Source: CAD feature listing. Evaluate the final solid. Frame: model axes, mm. Face numbers are marked on the shaded views. A direction names the side the tool comes from. Coordinates: 2 decimals unless noted, no trailing zeros. Loops run counter-clockwise (first coordinate to the right, second up) from the corner with the lowest first, then second, coordinate; pieces in that order, holes last. Notation, with made-up numbers: M 84.5,64 L 91.5,64 A22 ccw 91.5,75 Z; hole C -31,53.25 d6. An arc over 180 degrees is marked long. One line per question, with ' | ' between items. Start each with the question number.
1. Section query B-B, the plane x = 17.5. Output: boundary loops of the cut face in (y, z), and give its area (3 significant figures).
2. Section query A-A, the plane z = 3.5. Output: boundary loops of the cut face in (x, y), and give its area (3 significant figures).
3. Section query C-C, the plane y = 9.5. State how many separate pieces and enclosed holes the cut face has, and give its area (3 significant figures).
4. Ray query, probe 1 along Z at (x, y) = (17.5, 5.75); probe 2 along Z at (x, y) = (17.5, 2.1); probe 3 along X at (y, z) = (8, 3). Return the intervals inside material, ascending.
5. Mould query, pull axis X, two halves, no side actions, for the marked faces 1, 2, 3 and 4. Classes: pulls with the +X half, pulls with the -X half, needs draft (parallel to the pull), parting line crosses it, or undercut.
6. Access query for the marked faces 5 and 6. Directions: +Z, -Z, +X, -X, +Y, -Y. A direction counts if a zero-diameter tool reaches every point of the face in a straight line with its end or side. Return the directions, or none.
7. Section query D-D, the plane z = 22.5. Output: boundary loops of the cut face in (x, y).
8. Pin query (flat end, axial travel): P1, Ø12, axis at y = 15, z = 16.5, coming from the +X side; P2, Ø1.8, axis at x = 19, y = 8.5, coming from the +Z side; P3, Ø6, axis at x = 18, z = 9.5, coming from the +Y side. Return the tip coordinate at first contact, or that it passes through.
```python
from build123d import *

# Parameters (mm, degrees)
F0_W      = 20
F0_H      = 20
F0_R      = 2.75
F1_DEPTH  = 4
F2_W      = 20
F2_H      = 26
F3_DEPTH  = 3
F5_W      = 5
F5_H      = 9
F6_DEPTH  = 3
F4_R      = 1.4
F7_DEPTH  = 10
F9_DEPTH  = 3
F10_SIZE2 = 1.49999
F10_SIZE  = 2.99999


# Not quite as in the source:
# - a fillet or chamfer is up to 0.001 mm smaller than in the source, because OpenCascade refuses the exact size


with BuildPart() as f1:
    # F0 (on Top) → F1 (new body)
    with BuildSketch(Plane.XY):
        with Locations((10, 10)):
            Rectangle(F0_W, F0_H)
        with Locations((10, 10)):
            Circle(F0_R, mode=Mode.SUBTRACT)
    extrude(amount=F1_DEPTH)

    # F2 (on face) → F3 (join)
    with BuildSketch(Plane.XZ):
        with Locations((10, 13)):
            Rectangle(F2_W, F2_H)
    extrude(amount=-F3_DEPTH)

    # F5 (on face) → F6 (join)
    with BuildSketch(Plane.XY.offset(4)):
        with Locations((17.5, 7.5)):
            Rectangle(F5_W, F5_H)
    extrude(amount=F6_DEPTH)

    # F4 (on face) → F7 (cut)
    with BuildSketch(Plane.XZ):
        with Locations((17.5, 3.5)):
            Circle(F4_R)
        with Locations((17.5, 22.5)):
            Circle(F4_R)
    extrude(amount=-F7_DEPTH, mode=Mode.SUBTRACT)

    # F8 (on face) → F9 (join)
    with BuildSketch(Plane(origin=(0, 0, 0), x_dir=(0, -1, 0), z_dir=(-1, 0, 0))):
        Polygon((-3, 4), (-3, 26), (-20, 4), align=None)
    extrude(amount=-F9_DEPTH)

    # F10 (size 3 and 1.5 in the source; OpenCascade refuses exactly that, so slightly less here)
    f10_edges = [f1.edges().sort_by_distance(p)[0] for p in [
        (15, 7.5, 7),
    ]]
    f10_side = f1.faces().sort_by_distance((15, 7.5, 5.5))[0]
    chamfer(f10_edges, length=F10_SIZE, length2=F10_SIZE2, reference=f10_side)


solid = f1.part
```
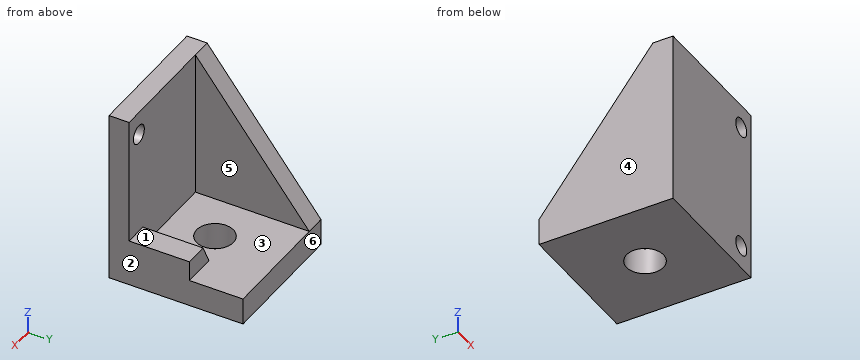
Taken from the geometry:
1) outline: M 0,0 L 20,0 L 20,4 L 12,4 L 12,7 L 3,7 L 3,21.1 L 0,21.1 L 0,4.9 L 10,4.9 L 10,2.1 L 0,2.1 Z; M 0,23.9 L 3,23.9 L 3,26 L 0,26 Z | area: 137 mm^2
2) outline: M 0,0 L 16.1,0 L 16.1,10 L 18.9,10 L 18.9,0 L 20,0 L 20,20 L 0,20 Z; hole C 10,10 d5.5 | area: 348 mm^2
3) separate pieces: 2 | enclosed holes: 1 | area: 106 mm^2
4) probe 1: 0 to 2.1, 4.9 to 7 | probe 2: 0 to 2.1, 4.9 to 21.1, 23.9 to 26 | probe 3: 0 to 8.11, 11.89 to 16.19, 18.81 to 20
5) face 1: needs draft | face 2: pulls with the +X half | face 3: undercut | face 4: pulls with the -X half
6) face 5: +Z, +Y | face 6: +Z, -Z, +X, -X, +Y
7) outline: M 0,0 L 16.1,0 L 16.1,3 L 3,3 L 3,5.7 L 0,5.7 Z; M 18.9,0 L 20,0 L 20,3 L 18.9,3 Z
8) P1: x = 3 | P2: z = 7 | P3: y = 12
